Here's the drawing with two shaded views (mm, measured from the low corner). I have some questions. A direction names the side the tool comes from. Give positions to 0.01 mm unless a question says otherwise; leave off trailing zeros. Loops run counter-clockwise (first coordinate to the right, second up) from the corner with the lowest first, then second, coordinate; pieces in that order, holes last. Notation, with made-up numbers: (54.5, -27) -> (98.5, -27) arc R18 ccw to (98.5, 8) -> close; hole circle Ø7 at (40.25, 30.25). An arc over 180 degrees is marked (long way). Answer in a Markdown table with one row per item. Add a question column.
Item 1: For P1, Ø1.5, axis at x = 14.5, y = 21.5, coming from the +Z side; P2, Ø9.5, axis at x = 12, z = 26, coming from the +Y side; P3, Ø6.5, axis at x = 20.5, y = 4, coming from the +Z side, each with a flat end and sliding along its axis, tell me the tip position at first contact or that it passes through.
Item 2: We'd pull the mould along X, two halves only. Please class the marked faces 1, 2 and 3: released by +X, released by -X, zero draft, split by the parting line, or undercut.
Item 3: If we section it at B-B (y = 2): Write out the boundary of the cut face in (x, z), then the cut area to 3 significant figures.
Item 4: If I drill on line 1 (Z direction, x = 24, y = 21.75); line 2 (Z direction, x = 13, y = 2.75), over which ranges is the centre line in solid material (lowest first)?
Item 5: If we section it at C-C (x = 4.5): Write out the boundary of the cut face in (y, z), then the cut area to 4 significant figures.
Item 6: If we section it at A-A (z = 21.5): Write out the boundary of the cut face in (x, y).
Item 7: If we section it at D-D (x = 18.5): Write out the boundary of the cut face in (y, z), then the cut area to 3 significant figures.
Item 8: Which directions (+Z, -Z, +X, -X, +Y, -Y) give clear straight access to the entire face, cutting with the end or side of a thin tool? Please do the marked faces 4, 5 and 6.
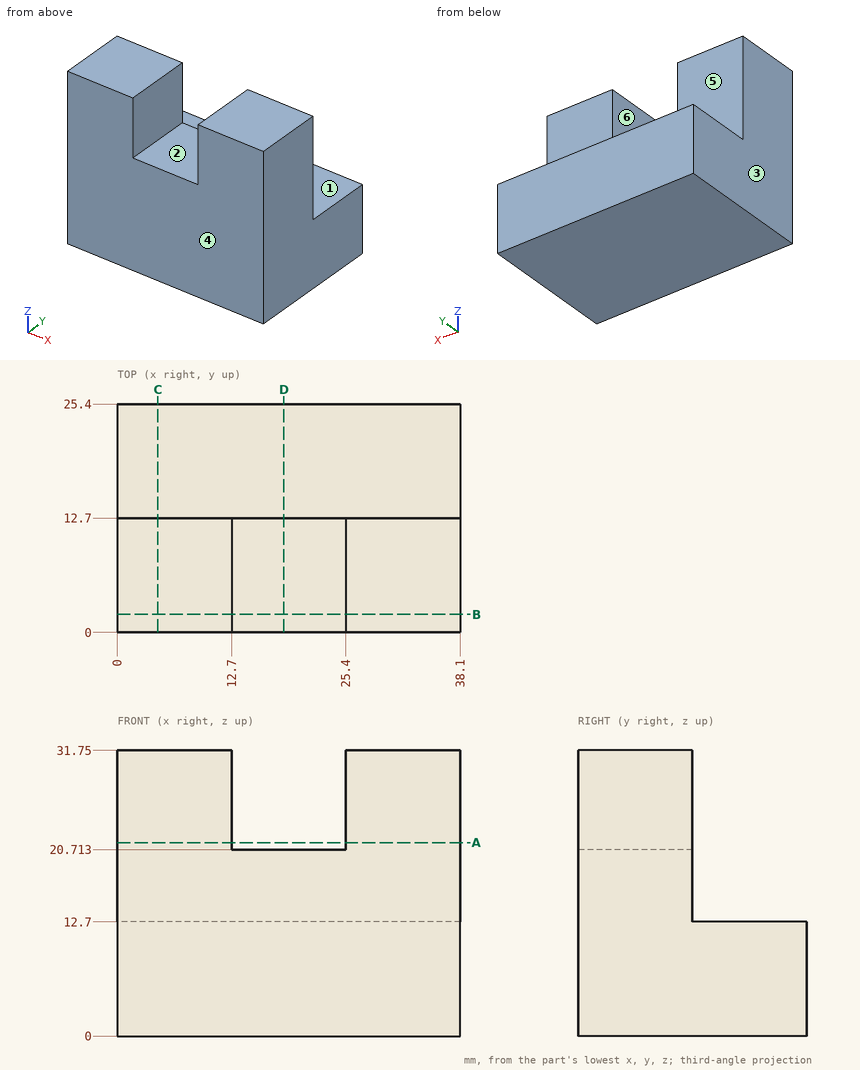
Recorded:
| question | item | result |
|---|---|---|
| 1 | P1 | stops at z = 12.7 |
| 1 | P2 | stops at y = 12.7 |
| 1 | P3 | stops at z = 20.71 |
| 2 | face 1 | zero draft |
| 2 | face 2 | undercut |
| 2 | face 3 | released by -X |
| 3 | outline | (0, 0) -> (38.1, 0) -> (38.1, 31.75) -> (25.4, 31.75) -> (25.4, 20.71) -> (12.7, 20.71) -> (12.7, 31.75) -> (0, 31.75) -> close |
| 3 | area | 1,070 mm^2 |
| 4 | line 1 | z = 0 to 12.7 |
| 4 | line 2 | z = 0 to 20.71 |
| 5 | outline | (0, 0) -> (25.4, 0) -> (25.4, 12.7) -> (12.7, 12.7) -> (12.7, 31.75) -> (0, 31.75) -> close |
| 5 | area | 564.5 mm^2 |
| 6 | outline | (0, 0) -> (12.7, 0) -> (12.7, 12.7) -> (0, 12.7) -> close; (25.4, 0) -> (38.1, 0) -> (38.1, 12.7) -> (25.4, 12.7) -> close |
| 7 | outline | (0, 0) -> (25.4, 0) -> (25.4, 12.7) -> (12.7, 12.7) -> (12.7, 20.71) -> (0, 20.71) -> close |
| 7 | area | 424 mm^2 |
| 8 | face 4 | +Z, -Z, +X, -X, -Y |
| 8 | face 5 | +Z, +X, -X, +Y |
| 8 | face 6 | +Z, +Y, -Y |
